```python
from build123d import *

# Parameters (mm, degrees)
SKETCH1_R           = 5
SKETCH1_R_2         = 2.78
BOSS_EXTRUDE1_DEPTH = 100
SKETCH2_W           = 20
SKETCH2_H           = 20
BOSS_EXTRUDE2_DEPTH = 20


with BuildPart() as part:
    # Sketch1 → Boss-Extrude1 (new body)
    with BuildSketch(Plane(origin=(0, 0, 0), x_dir=(1, 0, 0), z_dir=(0, 1, 0))):
        with Locations(Location((0, 0, 0), (0, 0, 270))):
            Circle(SKETCH1_R)
        with Locations(Location((0, 0, 0), (0, 0, 270))):
            Circle(SKETCH1_R_2, mode=Mode.SUBTRACT)
    extrude(amount=BOSS_EXTRUDE1_DEPTH)

    # Sketch2 → Boss-Extrude2 (add)
    with BuildSketch(Plane.XZ):
        Rectangle(SKETCH2_W, SKETCH2_H)
    extrude(amount=BOSS_EXTRUDE2_DEPTH)


solid = part.part
```
The model under review builds one solid part; all positions refer to its coordinate system, in mm. A direction names the side the tool comes from. Round coordinates to 2 decimals unless told otherwise and drop trailing zeros. Write each loop counter-clockwise with the first axis right and the second up, starting at its lowest first coordinate (ties: lowest second). Pieces come first, ordered by that corner, then holes.
(1) Machinability: for faces 1 (the flat face through (-2.2, 100, 2.2)), 2 (the flat face through (-2, 0, 5)), which of the approach directions +Z, -Z, +X, -X, +Y, -Y give a long, thin tool a straight path to every point of the face, cutting with its end or side? Answer none if there is none.
(2) We need section A-A on z = 0. Give the boundary of the cut face in (x, y), and give its area (3 significant figures).
(3) Mouldability with a two-part tool opening along X and no side actions: class faces 3 (the flat face through (0, 0, 0)), 4 (the cylindrical face through (-4.88, 49.3, -1.08)), 5 (the flat face through (0, -10, -10)) as +X half, -X half, draft (parallel to the pull), parting line (faces both ways), or undercut.
(4) Insertion check: pin 1 (3 mm diameter, centred on y = 12, z = -3, fed in from +X); pin 2 (4 mm diameter, centred on y = 48, z = -5, fed in from +X); pin 3 (1 mm diameter, centred on x = 7.5, z = 1, fed in from +Y); pin 4 (2 mm diameter, centred on y = 66, z = 7, fed in from -X). Each pin has a flat end and moves straight along its axis. Give the tip position at first contact, or say it passes through.
(5) Wall thickness on L1, parallel to X at y = 60.5, z = 0; L2, parallel to Y at x = -4.75, z = 2.5; L3, parallel to Z at x = -2.5, y = 13.5: over which ranges is each line inside the solid? List them lowest first.
(6) We need section B-B on y = 18. Give the boundary of the cut face in (x, z), and give its area (3 significant figures).
(7) We need section C-C on x = 0. Give the boundary of the cut face in (y, z), and give its area (3 significant figures).
(8) We need section D-D on z = 6. Give the boundary of the cut face in (x, y).
Findings below:
1. face 1: +Z, -Z, +X, -X, +Y
1. face 2: +Y
2. outline: (-10, -20) - (10, -20) - (10, 0) - (5, 0) - (5, 100) - (2.78, 100) - (2.78, 0) - (-2.78, 0) - (-2.78, 100) - (-5, 100) - (-5, 0) - (-10, 0) - close
2. area: 844 mm2
3. face 3: undercut
3. face 4: parting line
3. face 5: draft
4. pin 1: stops at x = 4.77
4. pin 2: stops at x = 4
4. pin 3: stops at y = 0
4. pin 4: passes through
5. L1: x = -5 to -2.78, 2.78 to 5
5. L2: y = -20 to 0
5. L3: z = -4.33 to -1.22, 1.22 to 4.33
6. outline: circle Ø10 at (0, 0); hole circle Ø5.56 at (0, 0)
6. area: 54.3 mm2
7. outline: (-20, -10) - (0, -10) - (0, -5) - (100, -5) - (100, -2.78) - (0, -2.78) - (0, 2.78) - (100, 2.78) - (100, 5) - (0, 5) - (0, 10) - (-20, 10) - close
7. area: 844 mm2
8. outline: (-10, -20) - (10, -20) - (10, 0) - (-10, 0) - close
